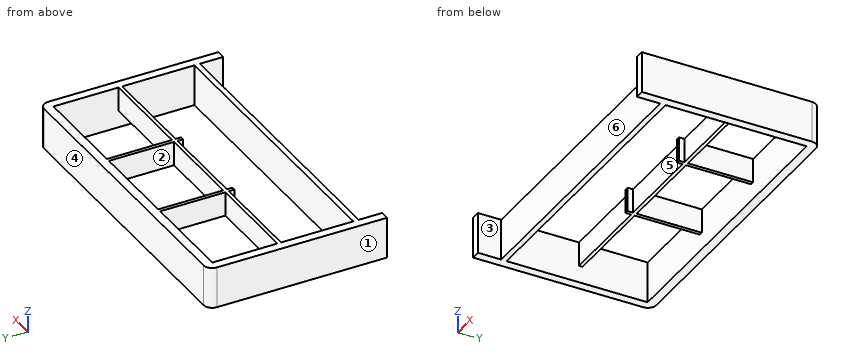
Autodesk Inventor part; units mm, degrees
ref_plane "YZ Plane" through (0, 0, 0) normal (1, 0, 0) x (0, 1, 0)
ref_plane "XZ Plane" through (0, 0, 0) normal (0, 1, 0) x (-1, 0, 0)
ref_plane "XY Plane" through (0, 0, 0) normal (0, 0, 1) x (1, 0, 0)
ref_plane "boardTop(tolerance)" through (29.1257, 19.6924, 40.7272) normal (0, -1, 0) x (1, 0, 0)
sketch "Sketch3" plane through (29.1257, 19.6924, 40.7272) normal (0, -1, 0) x (1, 0, 0)
  line L0 (-2, 1.51) -> (-2, 0)
  line L1 (158.35, 0) -> (158.35, 1.51)
  line L2 (-8, 18.0177) -> (-8, -5)
  line L3 (164.35, 18.0177) -> (164.35, -5)
  line L4 (164.35, 18.0177) -> (-8, 18.0177)
  line L5 (-8, -5) -> (164.35, -5)
  point P0 (-29.1257, -40.7272)
  point P1 (158.35, 0.755)
  dimension "d12" = 6
  dimension "d13" = 6
extrude "Extrusion3" add sketch "Sketch3" against normal blind 5
ref_plane "boardBottom(tolerance)" through (185.4757, -59.8376, 42.2372) normal (0, -1, 0) x (-1, 0, 0)
sketch "Sketch4" plane through (29.1257, 19.6924, 40.7272) normal (0, -1, 0) x (1, 0, 0)
  line L0 (-2, 1.51) -> (-2, 0)
  line L1 (158.35, 1.51) -> (158.35, 0)
  line L2 (-8, 18.0177) -> (-8, -5)
  line L3 (-8, -5) -> (164.35, -5)
  line L4 (164.35, -5) -> (164.35, 18.0177)
  line L5 (164.35, 18.0177) -> (-8, 18.0177)
  line L6 (159.35, -5) -> (159.35, 18.0177)
  line L7 (-8, 18.0177) -> (164.35, 18.0177)
  line L8 (-3, -5) -> (-3, 18.0177)
  point P0 (-29.1257, -40.7272)
  point P1 (158.35, 0.755)
  point P2 (-2, 0.755)
  point P3 (-3, 18.0177)
  dimension "d17" = 1
  dimension "d18" = 1
extrude "Extrusion4" add sketch "Sketch4" along normal blind 94.5274 contours L5 L8 L3 L2 | L5 L4 L3 L6
ref_plane "boardRight(tolerance)" through (188.4757, 19.6924, 35.7272) normal (-1, 0, 0) x (0, -1, 0)
sketch "Sketch5" plane through (188.4757, -74.835, 35.7272) normal (-1, 0, 0) x (0, 0, 1)
  line L0 (5, 15.9974) -> (6.51, 15.9974)
  line L1 (0, 94.5274) -> (23.0177, 94.5274)
  line L2 (0, 94.5274) -> (0, 0)
  line L3 (23.0177, 0) -> (0, 0)
  line L4 (23.0177, 94.5274) -> (23.0177, 0)
  line L5 (0, 94.5274) -> (0, 0)
  line L6 (0, 15.9974) -> (23.0177, 15.9974)
  line L7 (23.0177, 15.9974) -> (23.0177, 12.9974)
  line L8 (23.0177, 12.9974) -> (0, 12.9974)
  line L9 (0, 12.9974) -> (0, 15.9974)
  point P0 (-35.7272, 74.835)
  point P1 (0, 12.9974)
  point P2 (6.51, 15.9974)
  dimension "d21" = 3
ref_plane "boardLeft(tolerance)" through (26.1257, 19.6924, 58.7449) normal (1, 0, 0) x (0, -1, 0)
extrude "Extrusion5" add sketch "Sketch5" along normal up to surface (162.35 mm away) contours L0 L6 L4 L8 L2
sketch "Sketch6" plane through (29.1257, 19.6924, 40.7272) normal (0, -1, 0) x (1, 0, 0)
  line L0 (48.3131, 6.295) -> (48.54, 4.395)
  line L1 (54.3069, 2.495) -> (54.08, 4.395)
  line L2 (99.8531, 6.295) -> (100.08, 4.395)
  line L3 (107.5969, 2.495) -> (107.37, 4.395)
  line L4 (-3, 18.0177) -> (-3, -5)
  line L5 (-3, -5) -> (159.35, -5)
  line L6 (159.35, -5) -> (159.35, 18.0177)
  line L7 (159.35, 18.0177) -> (-3, 18.0177)
  line L8 (0, 1.51) -> (156.35, 1.51)
  line L9 (102.725, 1.51) -> (104.725, 1.51)
  line L10 (104.725, 1.51) -> (104.725, 18.0177)
  line L11 (104.725, 18.0177) -> (102.725, 18.0177)
  line L12 (102.725, 18.0177) -> (102.725, 1.51)
  line L13 (159.35, 18.0177) -> (-3, 18.0177)
  line L14 (50.31, 1.51) -> (52.31, 1.51)
  line L15 (52.31, 1.51) -> (52.31, 18.0177)
  line L16 (52.31, 18.0177) -> (50.31, 18.0177)
  line L17 (50.31, 18.0177) -> (50.31, 1.51)
  line L18 (48.4266, 5.345) -> (50.31, 5.345) construction
  line L19 (54.1934, 3.445) -> (52.31, 3.445) construction
  line L20 (99.9666, 5.345) -> (102.725, 5.345) construction
  line L21 (107.4834, 3.445) -> (104.725, 3.445) construction
  point P0 (-29.1257, -40.7272)
  point P1 (124.6421, 15.795)
  dimension "d31" = 2
  dimension "d32" = 2
extrude "Extrusion6" add sketch "Sketch6" along normal blind 41.275 contours L7 L15 L8 L17 | L7 L10 L8 L12
sketch "Sketch7" plane through (133.8507, 19.6924, 42.2372) normal (0, 0, -1) x (-1, 0, 0)
  line L0 (2, 0) -> (2, -41.275)
  line L1 (0, 0) -> (0, -41.275)
  line L2 (2, -41.275) -> (0, -41.275)
  line L3 (54.415, 0) -> (54.415, -41.275)
  line L4 (52.415, 0) -> (52.415, -41.275)
  line L5 (54.415, -41.275) -> (52.415, -41.275)
  line L6 (0, 0) -> (2, 0)
  line L7 (54.415, 0) -> (52.415, 0)
  point P0 (133.8507, -19.6924)
extrude "Extrusion7" cut sketch "Sketch7" against normal blind 3
sketch "Sketch9" plane through (188.4757, 19.6924, 35.7272) normal (-1, 0, 0) x (0, 0, 1)
  line L0 (23.0177, 0) -> (23.0177, -41.275)
  line L1 (23.0177, -41.275) -> (9.51, -41.275)
  line L2 (9.51, 0) -> (9.51, -41.275)
  line L3 (9.51, -38.275) -> (23.0177, -38.275)
  line L4 (23.0177, 0) -> (23.0177, -78.53)
  line L5 (9.51, -36.275) -> (23.0177, -36.275)
  point P0 (-35.7272, -19.6924)
  point P1 (23.0177, -36.275)
  point P2 (23.0177, -38.275)
  dimension "d35" = 3
  dimension "d37" = 2
extrude "Extrusion8" add sketch "Sketch9" along normal up to surface (162.35 mm away) contours L0 L3 L2 L5
fillet "Fillet1" radius 4.7625 2 edges at (21.1257, 24.6924, 47.236) (193.4757, 24.6924, 47.236)
properties part number "case"
Can you work these out from the model? Positions are in its coordinate system, mm. Face numbers are marked on the shaded views. A direction names the side the tool comes from. Round coordinates to 2 decimals unless told otherwise and drop trailing zeros. Write each loop counter-clockwise with the first axis right and the second up, starting at its lowest first coordinate (ties: lowest second). Pieces come first, ordered by that corner, then holes. Notation, with made-up numbers: (40.25, 23.5) - (65.25, 23.5) arc R22 cw to (65.25, 29.5) - close; hole circle Ø2 at (77, -2). An arc over 180 degrees is marked (long way). Write each question's results on one line, items separated by ' | '. Start each with the question number.
1) Suppose I cut it at B-B (y = -54.5). List the corners of the cut face in (x, z) for me, and give its area (3 significant figures).
2) Which directions (+Z, -Z, +X, -X, +Y, -Y) give clear straight access to the entire face, cutting with the end or side of a thin tool? Please do the marked faces 1, 2 and 3.
3) Suppose I cut it at A-A (x = 119). List the corners of the cut face in (y, z) for me, and give its area (3 significant figures).
4) For pin 1 Ø8 at (x, z) = (47, 48.5) entering from -Y, with a flat end and sliding along its axis, tell me the tip position at first contact or that it passes through.
5) We'd pull the mould along Y, two halves only. Please class the marked faces 4, 5 and 6: released by +Y, released by -Y, zero draft, split by the parting line, or undercut.
6) Suppose I cut it at C-C (z = 48.5). Give the number of separate pieces and of enclosed holes in the cut face, and give its area (3 significant figures).
7) Please list where these lines run through material, in increasing order: line 1 (Y direction, x = 46, z = 56.75); line 2 (X direction, y = -2, z = 50.5); line 3 (X direction, y = -5, z = 37.5).
Here are the results:
1) outline: (21.13, 35.73) - (26.13, 35.73) - (26.13, 58.74) - (21.13, 58.74) - close; (188.48, 35.73) - (193.48, 35.73) - (193.48, 58.74) - (188.48, 58.74) - close | area: 230 mm2
2) face 1: +Z, -Z, -X, +Y, -Y | face 2: +Z, -Z | face 3: +Z, -Z, -Y
3) outline: (-61.84, 35.73) - (-58.84, 35.73) - (-58.84, 58.74) - (-61.84, 58.74) - close; (-18.58, 45.24) - (-16.58, 45.24) - (-16.58, 58.74) - (-18.58, 58.74) - close; (19.69, 35.73) - (24.69, 35.73) - (24.69, 58.74) - (19.69, 58.74) - close | area: 211 mm2
4) pin 1: stops at y = -61.84
5) face 4: released by +Y | face 5: undercut | face 6: released by -Y
6) separate pieces: 1 | enclosed holes: 4 | area: 2,770 mm2
7) line 1: y = -61.84 to -58.84, -18.58 to -16.58, 19.69 to 24.69 | line 2: x = 21.13 to 26.13, 79.44 to 81.44, 131.85 to 133.85, 188.48 to 193.48 | line 3: x = 21.13 to 26.13, 188.48 to 193.48
